Design review of the part built by this model. Coordinates are the model's own, in mm. Coordinates: 2 decimals unless noted, no trailing zeros. Write each loop counter-clockwise with the first axis right and the second up, starting at its lowest first coordinate (ties: lowest second). Pieces come first, ordered by that corner, then holes. Notation, with made-up numbers: (18, -35) -> (66, -35) arc R21 cw to (66, -13) -> close; hole circle Ø4 at (-6, 64.5). An arc over 180 degrees is marked (long way). Answer in a Markdown table with one row per item. Add a question column.
Item 1: Take a section at A-A, the plane x = -36. Write out the cut boundary in (y, z), and give its area (3 significant figures).
Item 2: To check wall thickness, follow line 1 (X direction, y = 0.95, z = 10); line 2 (Z direction, x = -36, y = 1.8); line 3 (Z direction, x = -12, y = 1.7). State the ranges of each line that lie inside material, in increasing order.
Item 3: Take a section at B-B, the plane y = 0.8. Give the number of separate pieces and of enclosed holes in the cut face, and give its area (3 significant figures).
Item 4: Take a section at D-D, the plane x = 1. Write out the cut boundary in (y, z).
Item 5: Draft analysis for pull direction Z (two halves, no side actions). For faces 1 (the face through (48.196, 1.521, -33.289)), 2 (the face through (43.536, 1.479, -30.325)), 3 (the face through (50, 1, 21)), state which applies: released by +Z, released by -Z, zero draft, split by the parting line, or undercut.
Item 6: Clearance check with a flat-ended pin moving along its axis: P1, Ø5, axis at x = 20, z = 43.81, coming from the -Y side. State where the tip first meets the part, or that it passes through.
Item 7: Take a section at C-C, the plane z = 30. Write out the cut boundary in (x, y).
from build123d import *

# Parameters (mm, degrees)
SKETCH1_W           = 100
SKETCH1_H           = 70
BOSS_EXTRUDE1_DEPTH = 3
SKETCH2_R           = 1.5
CUT_EXTRUDE3_DEPTH  = 4
SKETCH3_W           = 50
SKETCH3_H           = 40
BOSS_EXTRUDE2_DEPTH = 3
CUT_EXTRUDE4_REACH  = 92.189
SKETCH4_R           = 1.5
SKETCH5_R           = 1.5
CUT_EXTRUDE5_DEPTH  = 3
CUT_EXTRUDE6_REACH  = 92.189
SKETCH6_R           = 1.5
CUT_EXTRUDE7_REACH  = 92.189
SKETCH8_R           = 1.5
SKETCH9_W           = 25
SKETCH9_H           = 40
SKETCH9_W_2         = 10.1139551
SKETCH9_H_2         = 8.275054173
BOSS_EXTRUDE3_DEPTH = 3
FILLET1_R           = 6


with BuildPart() as part:
    # Sketch1 → Boss-Extrude1 (new body)
    with BuildSketch(Plane(origin=(0, 0, 0), x_dir=(1, 0, 0), z_dir=(0, 1, 0))):
        Rectangle(SKETCH1_W, SKETCH1_H)
    extrude(amount=BOSS_EXTRUDE1_DEPTH)

    # Sketch2 → Cut-Extrude3 (cut)
    with BuildSketch(Plane(origin=(0, 0, 0), x_dir=(1, 0, 0), z_dir=(0, 1, 0))):
        with Locations(Location((-45, -30, 0), (0, 0, 270))):
            Circle(SKETCH2_R)
        with Locations(Location((45, -30, 0), (0, 0, 270))):
            Circle(SKETCH2_R)
        with Locations(Location((45, 30, 0), (0, 0, 270))):
            Circle(SKETCH2_R)
        with Locations(Location((-45, 30, 0), (0, 0, 270))):
            Circle(SKETCH2_R)
        with Locations(Location((-36, -20, 0), (0, 0, 270))):
            Circle(SKETCH2_R)
        with Locations(Location((36, -20, 0), (0, 0, 270))):
            Circle(SKETCH2_R)
        with Locations(Location((-36, -10, 0), (0, 0, 270))):
            Circle(SKETCH2_R)
        with Locations(Location((36, -10, 0), (0, 0, 270))):
            Circle(SKETCH2_R)
        with Locations(Location((-36, -15, 0), (0, 0, 270))):
            Circle(SKETCH2_R)
        with Locations(Location((36, -15, 0), (0, 0, 270))):
            Circle(SKETCH2_R)
    extrude(amount=CUT_EXTRUDE3_DEPTH, mode=Mode.SUBTRACT)

    # Sketch3 → Boss-Extrude2 (add)
    with BuildSketch(Plane(origin=(0, 0, 0), x_dir=(1, 0, 0), z_dir=(0, 1, 0))):
        with Locations((0, -55)):
            Rectangle(SKETCH3_W, SKETCH3_H)
    extrude(amount=BOSS_EXTRUDE2_DEPTH)

    # Sketch4 → Cut-Extrude4 (cut, up to next)
    with BuildSketch(Plane(origin=(0, 0, 0), x_dir=(1, 0, 0), z_dir=(0, 1, 0)), mode=Mode.PRIVATE) as cut_extrude4_sk1:
        with Locations(Location((-20, -70, 0), (0, 0, 90))):
            Circle(SKETCH4_R)
    cut_extrude4_tool1 = extrude(cut_extrude4_sk1.sketch, amount=CUT_EXTRUDE4_REACH, mode=Mode.PRIVATE) & part.part
    # Sketch4 → Cut-Extrude4 (cut, up to next)
    with BuildSketch(Plane(origin=(0, 0, 0), x_dir=(1, 0, 0), z_dir=(0, 1, 0)), mode=Mode.PRIVATE) as cut_extrude4_sk2:
        with Locations(Location((20, -70, 0), (0, 0, 90))):
            Circle(SKETCH4_R)
    cut_extrude4_tool2 = extrude(cut_extrude4_sk2.sketch, amount=CUT_EXTRUDE4_REACH, mode=Mode.PRIVATE) & part.part
    # Sketch4 → Cut-Extrude4 (cut, up to next)
    with BuildSketch(Plane(origin=(0, 0, 0), x_dir=(1, 0, 0), z_dir=(0, 1, 0)), mode=Mode.PRIVATE) as cut_extrude4_sk3:
        with Locations(Location((-20, -56, 0), (0, 0, 90))):
            Circle(SKETCH4_R)
    cut_extrude4_tool3 = extrude(cut_extrude4_sk3.sketch, amount=CUT_EXTRUDE4_REACH, mode=Mode.PRIVATE) & part.part
    # Sketch4 → Cut-Extrude4 (cut, up to next)
    with BuildSketch(Plane(origin=(0, 0, 0), x_dir=(1, 0, 0), z_dir=(0, 1, 0)), mode=Mode.PRIVATE) as cut_extrude4_sk4:
        with Locations(Location((20, -56, 0), (0, 0, 90))):
            Circle(SKETCH4_R)
    cut_extrude4_tool4 = extrude(cut_extrude4_sk4.sketch, amount=CUT_EXTRUDE4_REACH, mode=Mode.PRIVATE) & part.part
    # Sketch4 → Cut-Extrude4 (cut, up to next)
    with BuildSketch(Plane(origin=(0, 0, 0), x_dir=(1, 0, 0), z_dir=(0, 1, 0)), mode=Mode.PRIVATE) as cut_extrude4_sk5:
        with Locations(Location((1, -63, 0), (0, 0, 90))):
            Circle(SKETCH4_R)
    cut_extrude4_tool5 = extrude(cut_extrude4_sk5.sketch, amount=CUT_EXTRUDE4_REACH, mode=Mode.PRIVATE) & part.part
    add(cut_extrude4_tool1.solids().sort_by_distance((-20, 0, 70))[0], mode=Mode.SUBTRACT)
    add(cut_extrude4_tool2.solids().sort_by_distance((20, 0, 70))[0], mode=Mode.SUBTRACT)
    add(cut_extrude4_tool3.solids().sort_by_distance((-20, 0, 56))[0], mode=Mode.SUBTRACT)
    add(cut_extrude4_tool4.solids().sort_by_distance((20, 0, 56))[0], mode=Mode.SUBTRACT)
    add(cut_extrude4_tool5.solids().sort_by_distance((1, 0, 63))[0], mode=Mode.SUBTRACT)

    # Sketch5 → Cut-Extrude5 (cut)
    with BuildSketch(Plane.XZ):
        with Locations((68.9999632, 26.624996827)):
            Circle(SKETCH5_R)
    extrude(amount=-CUT_EXTRUDE5_DEPTH, mode=Mode.SUBTRACT)

    # Sketch6 → Cut-Extrude6 (cut, up to next)
    with BuildSketch(Plane.XZ, mode=Mode.PRIVATE) as cut_extrude6_sk1:
        with Locations(Location((-20, 63.563183916, 0), (0, 0, 270))):
            Circle(SKETCH6_R)
    cut_extrude6_tool1 = extrude(cut_extrude6_sk1.sketch, amount=-CUT_EXTRUDE6_REACH, mode=Mode.PRIVATE) & part.part
    # Sketch6 → Cut-Extrude6 (cut, up to next)
    with BuildSketch(Plane.XZ, mode=Mode.PRIVATE) as cut_extrude6_sk2:
        with Locations(Location((20, 63.563183916, 0), (0, 0, 270))):
            Circle(SKETCH6_R)
    cut_extrude6_tool2 = extrude(cut_extrude6_sk2.sketch, amount=-CUT_EXTRUDE6_REACH, mode=Mode.PRIVATE) & part.part
    # Sketch6 → Cut-Extrude6 (cut, up to next)
    with BuildSketch(Plane.XZ, mode=Mode.PRIVATE) as cut_extrude6_sk3:
        with Locations(Location((20, 43.808225194, 0), (0, 0, 270))):
            Circle(SKETCH6_R)
    cut_extrude6_tool3 = extrude(cut_extrude6_sk3.sketch, amount=-CUT_EXTRUDE6_REACH, mode=Mode.PRIVATE) & part.part
    # Sketch6 → Cut-Extrude6 (cut, up to next)
    with BuildSketch(Plane.XZ, mode=Mode.PRIVATE) as cut_extrude6_sk4:
        with Locations(Location((-20, 49.40580256, 0), (0, 0, 270))):
            Circle(SKETCH6_R)
    cut_extrude6_tool4 = extrude(cut_extrude6_sk4.sketch, amount=-CUT_EXTRUDE6_REACH, mode=Mode.PRIVATE) & part.part
    # Sketch6 → Cut-Extrude6 (cut, up to next)
    with BuildSketch(Plane.XZ, mode=Mode.PRIVATE) as cut_extrude6_sk5:
        with Locations(Location((-20, 43.808225194, 0), (0, 0, 270))):
            Circle(SKETCH6_R)
    cut_extrude6_tool5 = extrude(cut_extrude6_sk5.sketch, amount=-CUT_EXTRUDE6_REACH, mode=Mode.PRIVATE) & part.part
    # Sketch6 → Cut-Extrude6 (cut, up to next)
    with BuildSketch(Plane.XZ, mode=Mode.PRIVATE) as cut_extrude6_sk6:
        with Locations(Location((20, 49.40580256, 0), (0, 0, 270))):
            Circle(SKETCH6_R)
    cut_extrude6_tool6 = extrude(cut_extrude6_sk6.sketch, amount=-CUT_EXTRUDE6_REACH, mode=Mode.PRIVATE) & part.part
    add(cut_extrude6_tool1.solids().sort_by_distance((-20, 0, 63.563184))[0], mode=Mode.SUBTRACT)
    add(cut_extrude6_tool2.solids().sort_by_distance((20, 0, 63.563184))[0], mode=Mode.SUBTRACT)
    add(cut_extrude6_tool3.solids().sort_by_distance((20, 0, 43.808225))[0], mode=Mode.SUBTRACT)
    add(cut_extrude6_tool4.solids().sort_by_distance((-20, 0, 49.405803))[0], mode=Mode.SUBTRACT)
    add(cut_extrude6_tool5.solids().sort_by_distance((-20, 0, 43.808225))[0], mode=Mode.SUBTRACT)
    add(cut_extrude6_tool6.solids().sort_by_distance((20, 0, 49.405803))[0], mode=Mode.SUBTRACT)

    # Sketch8 → Cut-Extrude7 (cut, up to next)
    with BuildSketch(Plane(origin=(0, 0, 0), x_dir=(1, 0, 0), z_dir=(0, 1, 0)), mode=Mode.PRIVATE) as cut_extrude7_sk1:
        with Locations(Location((-12, -72, 0), (0, 0, 90))):
            Circle(SKETCH8_R)
    cut_extrude7_tool1 = extrude(cut_extrude7_sk1.sketch, amount=CUT_EXTRUDE7_REACH, mode=Mode.PRIVATE) & part.part
    # Sketch8 → Cut-Extrude7 (cut, up to next)
    with BuildSketch(Plane(origin=(0, 0, 0), x_dir=(1, 0, 0), z_dir=(0, 1, 0)), mode=Mode.PRIVATE) as cut_extrude7_sk2:
        with Locations(Location((14, -72, 0), (0, 0, 90))):
            Circle(SKETCH8_R)
    cut_extrude7_tool2 = extrude(cut_extrude7_sk2.sketch, amount=CUT_EXTRUDE7_REACH, mode=Mode.PRIVATE) & part.part
    add(cut_extrude7_tool1.solids().sort_by_distance((-12, 0, 72))[0], mode=Mode.SUBTRACT)
    add(cut_extrude7_tool2.solids().sort_by_distance((14, 0, 72))[0], mode=Mode.SUBTRACT)

    # Sketch9 → Boss-Extrude3 (add)
    with BuildSketch(Plane(origin=(0, 0, 0), x_dir=(1, 0, 0), z_dir=(0, 1, 0))):
        with Locations((37.5, -55)):
            Rectangle(SKETCH9_W, SKETCH9_H)
        with Locations((-37.5, -55)):
            Rectangle(SKETCH9_W, SKETCH9_H)
        with Locations((36.349588901, -26.811598528)):
            Rectangle(SKETCH9_W_2, SKETCH9_H_2)
    extrude(amount=BOSS_EXTRUDE3_DEPTH)

    # Fillet1
    fillet1_edges = [part.edges().sort_by_distance(p)[0] for p in [
        (50, 1.5, 75),
        (-50, 1.5, 75),
        (-50, 1.5, -35),
        (50, 1.5, -35),
    ]]
    fillet(fillet1_edges, radius=FILLET1_R)


solid = part.part
Answers:
| question | item | result |
|---|---|---|
| 1 | outline | (0, -35) -> (3, -35) -> (3, 8.5) -> (0, 8.5) -> close; (0, 11.5) -> (3, 11.5) -> (3, 13.5) -> (0, 13.5) -> close; (0, 16.5) -> (3, 16.5) -> (3, 18.5) -> (0, 18.5) -> close; (0, 21.5) -> (3, 21.5) -> (3, 75) -> (0, 75) -> close |
| 1 | area | 303 mm^2 |
| 2 | line 1 | x = -50 to -37.5, -34.5 to 34.5, 37.5 to 50 |
| 2 | line 2 | z = -35 to 8.5, 11.5 to 13.5, 16.5 to 18.5, 21.5 to 75 |
| 2 | line 3 | z = -35 to 70.5, 73.5 to 75 |
| 3 | separate pieces | 1 |
| 3 | enclosed holes | 23 |
| 3 | area | 10,800 mm^2 |
| 4 | outline | (0, -35) -> (3, -35) -> (3, 61.5) -> (0, 61.5) -> close; (0, 64.5) -> (3, 64.5) -> (3, 75) -> (0, 75) -> close |
| 5 | face 1 | released by -Z |
| 5 | face 2 | undercut |
| 5 | face 3 | zero draft |
| 6 | P1 | stops at y = 0 |
| 7 | outline | (-50, 0) -> (-46.5, 0) -> (-46.5, 3) -> (-50, 3) -> close; (-43.5, 0) -> (43.5, 0) -> (43.5, 3) -> (-43.5, 3) -> close; (46.5, 0) -> (50, 0) -> (50, 3) -> (46.5, 3) -> close |
